Check sheet for the modelled part. Datum: model origin and axes. Units: mm. Round coordinates to 2 decimals unless told otherwise and drop trailing zeros. Order: outer loops, then holes, each group sorted by start corner. A loop starts at its lowest first (then second) coordinate and runs counter-clockwise, first axis right, second up.
Q1. Scan lines: probe 1 along X at (y, z) = (-4.1, 6.25); probe 2 along Z at (x, y) = (-9.75, -0.2); probe 3 along Z at (x, y) = (-7, -3.9). Record each from-to range of solid material in increasing order.
Q2. Mould release check, pull along Z, two halves, no side actions. Record for faces 1 (the cylindrical face through (5.324, -2.535, 8.375)), 2 (the flat face through (-12.045, -2, 2)), 3 (the flat face through (-2, -2, -6.172)): +Z half, -Z half, draft (parallel to the pull), parting line (faces both ways), or undercut.
Q3. Depth check by flat-ended pin: P1, Ø4, axis at x = 3.98, z = 6.27, coming from the +Y side. Enter the tip coordinate at first touch or a pass-through.
Q4. Cross-section at A-A on z = 4.25. Record the cut outline in (x, y).
Q5. Cross-section at B-B on x = -9.5. Record the cut outline in (y, z).
Q6. Cross-section at C-C on y = -1.55. Record the cut outline in (x, z), then the cut area to 3 significant figures.
from build123d import *

# Parameters (mm, degrees)
F0_W     = 20.36
F0_H     = 16
F1_DEPTH = 5
F2_R     = 2.5
F3_DEPTH = 5.001
F4_R     = 2.5
F5_DEPTH = 5.001


with BuildPart() as f1:
    # F0 (on Front) → F1 (new body)
    with BuildSketch(Plane.XZ):
        with Locations((-1.864513, 1.827734)):
            Rectangle(F0_W, F0_H)
    extrude(amount=F1_DEPTH)

    # F2 (on face) → F3 (cut, through all)
    with BuildSketch(Plane.XZ.offset(5)):
        with Locations((-7.754513, -1.832266)):
            Circle(F2_R)
    extrude(amount=-F3_DEPTH, mode=Mode.SUBTRACT)

    # F4 (on face) → F5 (cut, through all)
    with BuildSketch(Plane.XZ.offset(5)):
        with Locations((3.979688, 6.266656)):
            Circle(F4_R)
    extrude(amount=-F5_DEPTH, mode=Mode.SUBTRACT)


solid = f1.part
Results found:
1. probe 1: x = -12.04 to 1.48, 6.48 to 8.32
1. probe 2: z = -6.17 to -3.34, -0.33 to 9.83
1. probe 3: z = -6.17 to -4.22, 0.55 to 9.83
2. face 1: undercut
2. face 2: draft
2. face 3: -Z half
3. P1: passes through
4. outline: (-12.04, -5) - (2.5, -5) - (2.5, 0) - (-12.04, 0) - close; (5.46, -5) - (8.32, -5) - (8.32, 0) - (5.46, 0) - close
5. outline: (-5, -6.17) - (0, -6.17) - (0, -3.62) - (-5, -3.62) - close; (-5, -0.04) - (0, -0.04) - (0, 9.83) - (-5, 9.83) - close
6. outline: (-12.04, -6.17) - (8.32, -6.17) - (8.32, 9.83) - (-12.04, 9.83) - close; hole circle Ø5 at (-7.75, -1.83); hole circle Ø5 at (3.98, 6.27)
6. area: 286 mm2
